The model under review builds one solid part; all positions refer to its coordinate system, in mm. A direction names the side the tool comes from. Coordinates: 2 decimals unless noted, no trailing zeros. Order: outer loops, then holes, each group sorted by start corner. A loop starts at its lowest first (then second) coordinate and runs counter-clockwise, first axis right, second up. Notation, with made-up numbers: (69.5, -15) -> (77.5, -15) arc R29 cw to (77.5, 8) -> close; hole circle Ø4 at (-12.75, 11.5). An arc over 180 degrees is marked (long way). Use CSV: the item, a comma, the result in double quotes. Start each with the question number.
```python
from build123d import *

# Parameters (mm, degrees)
F1_DEPTH = 50.8
F2_R     = 5.08
F3_R     = 5.08
F4_R     = 5.08
F5_R     = 5.08


with BuildPart() as f1:
    # F0 (on Front) → F1 (new body)
    with BuildSketch(Plane.XZ):
        with BuildLine():
            Line((0, 114.3), (0, 0))
            Line((0, 0), (63.5, 0))
            Line((63.5, 0), (63.5, 114.3))
            Line((63.5, 114.3), (44.45, 114.3))
            ThreePointArc((44.45, 114.3), (31.75, 101.6), (19.05, 114.3))
            Line((19.05, 114.3), (0, 114.3))
        make_face()
    extrude(amount=-F1_DEPTH)

    # F2
    f2_edges = [f1.edges().sort_by_distance(p)[0] for p in [
        (19.05, 25.4, 114.3),
    ]]
    fillet(f2_edges, radius=F2_R)

    # F3
    f3_edges = [f1.edges().sort_by_distance(p)[0] for p in [
        (44.45, 25.4, 114.3),
    ]]
    fillet(f3_edges, radius=F3_R)

    # F4
    f4_edges = [f1.edges().sort_by_distance(p)[0] for p in [
        (63.5, 25.4, 114.3),
    ]]
    fillet(f4_edges, radius=F4_R)

    # F5
    f5_edges = [f1.edges().sort_by_distance(p)[0] for p in [
        (0, 25.4, 114.3),
    ]]
    fillet(f5_edges, radius=F5_R)


solid = f1.part
```
Q1. Add section D-D, the plane x = 29.5. State the section outline as (y, z) points.
Q2. Add section C-C, the plane x = 36.5. State the section outline as (y, z) points, then the cut area to 3 significant figures.
Q3. Add section A-A, the plane z = 104. State the section outline as (x, y) points.
Q4. Add section B-B, the plane y = 42. State the section outline as (x, z) points.
Q5. Clearance check with flat-ended pins moving along their axes: pin 1 Ø6 at (x, y) = (25.5, 6) entering from +Z; pin 2 Ø1 at (x, y) = (35, 22) entering from +Z. State where each tip first meets the part, or that it passes through.
Q6. Draft analysis for pull direction X (two halves, no side actions). For faces 3 (the cylindrical face through (17.78, 25.76, 113.27)), 4 (the flat face through (63.5, 25, 54)), 5 (the flat face through (31, 25, 0)), 6 (the cylindrical face through (31.978, 25.044, 101.602)), state which applies: +X half, -X half, draft (parallel to the pull), parting line (faces both ways), or undercut.
Q7. For faces 1 (the cylindrical face through (45.72, 25.76, 113.27)), 2 (the flat face through (31, 50.8, 58)), list the 3-axis set-ups (+Z, -Z, +X, -X, +Y, -Y) from which the entire face can be reached by the end or side of a thin tool; tool diameter is ignored.
Q8. To check wall thickness, follow probe 1 along X at (y, z) = (16, 109); probe 2 along Z at (x, y) = (15, 31); probe 3 along Z at (x, y) = (31, 6.5). State the ranges of each line that lie inside material, in increasing order.
Answer block:
1,outline,"(0, 0) -> (50.8, 0) -> (50.8, 101.8) -> (0, 101.8) -> close"
2,outline,"(0, 0) -> (50.8, 0) -> (50.8, 102.52) -> (0, 102.52) -> close"
2,area,"5,210 mm²"
3,outline,"(0, 0) -> (24.32, 0) -> (24.32, 50.8) -> (0, 50.8) -> close; (39.18, 0) -> (63.5, 0) -> (63.5, 50.8) -> (39.18, 50.8) -> close"
4,outline,"(0, 0) -> (63.5, 0) -> (63.5, 109.22) arc R5.08 ccw to (58.42, 114.3) -> (48.79, 114.3) arc R5.08 ccw to (43.92, 110.67) arc R12.7 cw to (19.58, 110.67) arc R5.08 ccw to (14.71, 114.3) -> (5.08, 114.3) arc R5.08 ccw to (0, 109.22) -> close"
5,pin 1,"stops at z = 105.6"
5,pin 2,"stops at z = 102.17"
6,face 3,"undercut"
6,face 4,"+X half"
6,face 5,"draft"
6,face 6,"undercut"
7,face 1,"+Z, +Y, -Y"
7,face 2,"+Z, -Z, +X, -X, +Y"
8,probe 1,"x = 0 to 20.21, 43.29 to 63.5"
8,probe 2,"z = 0 to 114.29"
8,probe 3,"z = 0 to 101.62"
